Work out the finished part from the listing and answer in its coordinate system (mm). A direction names the side the tool comes from. Coordinates: 2 decimals unless noted, no trailing zeros. Order: outer loops, then holes, each group sorted by start corner. A loop starts at its lowest first (then second) coordinate and runs counter-clockwise, first axis right, second up. Notation, with made-up numbers: M 44.25,70.25 L 70.25,70.25 A16 ccw 70.25,76.25 Z; hole C 26,75 d1. An arc over 180 degrees is marked long. Answer in a Markdown table with one row per item. Add a question column.
Item 1: Consider line 1 (X direction, y = -5, z = -5); line 2 (Y direction, x = 0, z = 5.5); line 3 (Y direction, x = 2, z = -7.75). Determine where each line is inside the solid, lowest interval first. Write a range as from..to.
Item 2: The part is cut by section B-B (z = 6.5). Write down the section's boundary in (x, y), then the cut area to 3 significant figures.
Item 3: Which of the six approach directions +Z, -Z, +X, -X, +Y, -Y give full straight-line access (tool end or side, diameter ignored) to faces 4 (the face through (4.867, 8.275, -6.056)), 5 (the face through (-6, 8, -10)), 6 (the face through (4.867, 8.275, 5.944))?
Item 4: Flat-ended cylindrical pins translate along their axes: pin 1 Ø1 at (x, z) = (-2.5, 7) entering from -Y; pin 2 Ø6 at (x, y) = (0, -3.5) entering from +Z; pin 3 Ø10 at (x, z) = (-8, -2.5) entering from -Y. Find the tip coordinate at first contact, or state that the pin passes through.
Item 5: The mould has two halves that part along X. Classify faces 1 (the face through (-6, 8, 10)), 2 (the face through (0, 0, -2)), 3 (the face through (-13.1, 0, 0)): released by +X, released by -X, zero draft, split by the parting line, or undercut.
Item 6: The part is cut by section A-A (y = -4.5). Write down the section's boundary in (x, z).
Item 7: The part is cut by section D-D (z = 1.25). Write down the section's boundary in (x, y), then the cut area to 3 significant figures.
Item 8: The part is cut by section C-C (x = -6.5). Write down the section's boundary in (y, z), then the cut area to 3 significant figures.
from build123d import *

# Parameters (mm, degrees)
BOSS_EXTRUDE1_DEPTH      = 10
BOSS_EXTRUDE1_DEPTH_BACK = 10
BOSS_EXTRUDE2_DEPTH      = 2
BOSS_EXTRUDE2_DEPTH_BACK = 2


with BuildPart() as part:
    # Sketch1 → Boss-Extrude1 (new, two sides: drawn at the far end of the back side and taken through both)
    with BuildSketch(Plane(origin=(0, 0, 0), x_dir=(0, 1, 0), z_dir=(0, 0, 1)).offset(-BOSS_EXTRUDE1_DEPTH_BACK)):
        Polygon((7.563288526, 13.1), (-7.563288526, 13.1), (-15.126577053, 0), (-7.563288526, -13.1), (7.563288526, -13.1), (15.126577053, 0), align=None)
        Polygon((5.542562584, 9.6), (-5.542562584, 9.6), (-11.085125168, 0), (-5.542562584, -9.6), (5.542562584, -9.6), (11.085125168, 0), align=None, mode=Mode.SUBTRACT)
    extrude(amount=BOSS_EXTRUDE1_DEPTH + BOSS_EXTRUDE1_DEPTH_BACK)

    # Sketch2 → Boss-Extrude2 (add, two sides: drawn at the far end of the back side and taken through both)
    with BuildSketch(Plane(origin=(0, 0, 0), x_dir=(0, 1, 0), z_dir=(0, 0, 1)).offset(-BOSS_EXTRUDE2_DEPTH_BACK)):
        Polygon((15.126577053, 0), (7.563288526, 13.1), (-7.563288526, 13.1), (-15.126577053, 0), (-7.563288526, -13.1), (7.563288526, -13.1), align=None)
    extrude(amount=BOSS_EXTRUDE2_DEPTH + BOSS_EXTRUDE2_DEPTH_BACK)


solid = part.part
Reply:
| question | item | result |
|---|---|---|
| 1 | line 1 | x = -13.1..-9.6, 9.6..13.1 |
| 1 | line 2 | y = -15.13..-11.09, 11.09..15.13 |
| 1 | line 3 | y = -13.97..-9.93, 9.93..13.97 |
| 2 | outline | M -13.1,-7.56 L 0,-15.13 L 13.1,-7.56 L 13.1,7.56 L 0,15.13 L -13.1,7.56 Z; hole M -9.6,-5.54 L 0,-11.09 L 9.6,-5.54 L 9.6,5.54 L 0,11.09 L -9.6,5.54 Z |
| 2 | area | 275 mm2 |
| 3 | face 4 | -Z |
| 3 | face 5 | -Z, +X, -X, +Y, -Y |
| 3 | face 6 | +Z |
| 4 | pin 1 | stops at y = -13.97 |
| 4 | pin 2 | stops at z = 2 |
| 4 | pin 3 | stops at y = -13.39 |
| 5 | face 1 | zero draft |
| 5 | face 2 | undercut |
| 5 | face 3 | released by -X |
| 6 | outline | M -13.1,-10 L -9.6,-10 L -9.6,-2 L 9.6,-2 L 9.6,-10 L 13.1,-10 L 13.1,10 L 9.6,10 L 9.6,2 L -9.6,2 L -9.6,10 L -13.1,10 Z |
| 7 | outline | M -13.1,-7.56 L 0,-15.13 L 13.1,-7.56 L 13.1,7.56 L 0,15.13 L -13.1,7.56 Z |
| 7 | area | 594 mm2 |
| 8 | outline | M -11.37,-10 L -7.33,-10 L -7.33,-2 L 7.33,-2 L 7.33,-10 L 11.37,-10 L 11.37,10 L 7.33,10 L 7.33,2 L -7.33,2 L -7.33,10 L -11.37,10 Z |
| 8 | area | 220 mm2 |
